Build history of the part. All positions in model axes, mm. Face numbers are marked on the shaded views. A direction names the side the tool comes from. Give positions to 0.01 mm unless a question says otherwise; leave off trailing zeros. Write each loop counter-clockwise with the first axis right and the second up, starting at its lowest first coordinate (ties: lowest second). Pieces come first, ordered by that corner, then holes. Notation, with made-up numbers: (45.25, 23.5) -> (60.25, 23.5) arc R24 cw to (60.25, 46.5) -> close; hole circle Ø4 at (-30.75, 31). An arc over 180 degrees is marked (long way). One line per question, with ' | ' between items. Start each with the question number.
(1) Drill centre lines: probe 1 along Z at (x, y) = (0, 2.6); probe 2 along Z at (x, y) = (0, 0.95); probe 3 along Y at (x, z) = (0.75, -2.75). Where is each one in solid material? Low to high. Write a range as from..to.
(2) Band-saw the part on B-B, the plane x = 2. Give the cut face in (y, z), and give its area (3 significant figures).
(3) Band-saw the part on D-D, the plane y = 9.25. Give the cut face in (x, z), and give its area (3 significant figures).
(4) Band-saw the part on A-A, the plane z = 0. Give the cut face in (x, y).
(5) Pull direction Z, two halves, no side cores. Call the marked faces 1, 2 and 3: released by +Z, released by -Z, zero draft, split by the parting line, or undercut.
(6) Tool access for the marked faces 4 and 5: list every direction of +Z, -Z, +X, -X, +Y, -Y with a clear straight run to the whole face (end or side of a thin tool).
(7) Pin check, flat tips, straight feed: P1, Ø5, axis at x = 2.5, y = 2, coming from the +Z side; P2, Ø3, axis at x = -0.5, z = -0.5, coming from the -Y side; P3, Ø2, axis at y = 5, z = -3, coming from the -X side. Stop position of each tip, or through.
(8) Band-saw the part on C-C, the plane y = 2.5. Give the cut face in (x, z).
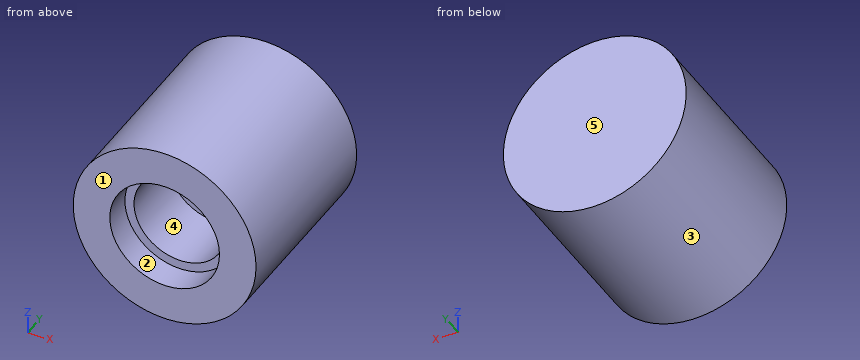
from build123d import *

# Parameters (mm, degrees)
SKETCH1_R           = 5
BOSS_EXTRUDE1_DEPTH = 10
SKETCH2_R           = 2.5
CUT_EXTRUDE1_DEPTH  = 5
SKETCH3_R           = 3
CUT_EXTRUDE2_DEPTH  = 1.5


with BuildPart() as part:
    # Sketch1 → Boss-Extrude1 (new body)
    with BuildSketch(Plane(origin=(0, 0, 0), x_dir=(1, 0, 0), z_dir=(0, 1, 0))):
        Circle(SKETCH1_R)
    extrude(amount=BOSS_EXTRUDE1_DEPTH)

    # Sketch2 → Cut-Extrude1 (cut)
    with BuildSketch(Plane.XZ):
        Circle(SKETCH2_R)
    extrude(amount=-CUT_EXTRUDE1_DEPTH, mode=Mode.SUBTRACT)

    # Sketch3 → Cut-Extrude2 (cut)
    with BuildSketch(Plane.XZ):
        Circle(SKETCH3_R)
    extrude(amount=-CUT_EXTRUDE2_DEPTH, mode=Mode.SUBTRACT)


solid = part.part
Results:
1) probe 1: z = -5..-2.5, 2.5..5 | probe 2: z = -5..-3, 3..5 | probe 3: y = 1.5..10
2) outline: (0, -4.58) -> (10, -4.58) -> (10, 4.58) -> (0, 4.58) -> (0, 2.24) -> (1.5, 2.24) -> (1.5, 1.5) -> (5, 1.5) -> (5, -1.5) -> (1.5, -1.5) -> (1.5, -2.24) -> (0, -2.24) -> close | area: 74.4 mm²
3) outline: circle Ø10 at (0, 0) | area: 78.5 mm²
4) outline: (-5, 0) -> (-3, 0) -> (-3, 1.5) -> (-2.5, 1.5) -> (-2.5, 5) -> (2.5, 5) -> (2.5, 1.5) -> (3, 1.5) -> (3, 0) -> (5, 0) -> (5, 10) -> (-5, 10) -> close
5) face 1: zero draft | face 2: undercut | face 3: split by the parting line
6) face 4: -Y | face 5: +Z, -Z, +X, -X, +Y
7) P1: stops at z = 5 | P2: stops at y = 5 | P3: stops at x = -4.58
8) outline: circle Ø10 at (0, 0); hole circle Ø5 at (0, 0)
